The model under review builds one solid part; all positions refer to its coordinate system, in mm. Face numbers are marked on the shaded views. A direction names the side the tool comes from. Round coordinates to 2 decimals unless told otherwise and drop trailing zeros. Loops run counter-clockwise (first coordinate to the right, second up) from the corner with the lowest first, then second, coordinate; pieces in that order, holes last. Notation, with made-up numbers: M 17,83.5 L 36,83.5 A19 cw 36,94.5 Z; hole C 45,57 d10. An arc over 180 degrees is marked long. One line per question, with ' | ' between items.
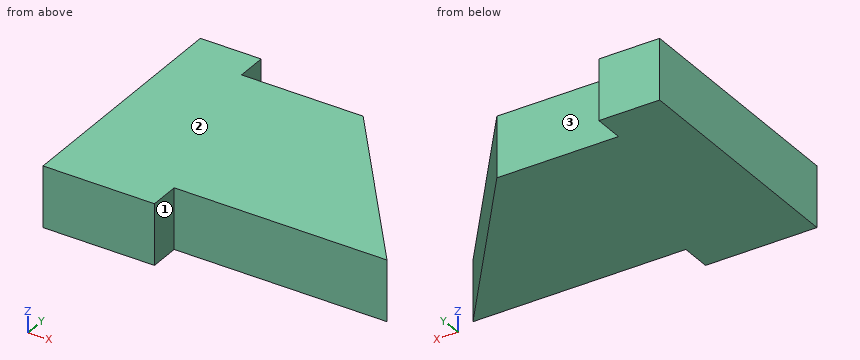
from build123d import *

# Parameters (mm, degrees)
EXTRUDE_1_DEPTH = 3
SKETCH_2_W      = 3
SKETCH_2_H      = 3
EXTRUDE_2_DEPTH = 1.5
SKETCH_3_W      = 5.5
SKETCH_3_H      = 3
EXTRUDE_3_DEPTH = 1.5


with BuildPart() as part:
    # Эскиз1 → Бобышка-Вытянуть1 (new body)
    with BuildSketch(Plane.XY):
        Polygon((0, 9), (0, 0), (16, 0), (9, 9), align=None)
    extrude(amount=EXTRUDE_1_DEPTH)

    # Эскиз2 → Бобышка-Вытянуть2 (add)
    with BuildSketch(Plane(origin=(0, 9, 0), x_dir=(1, 0, 0), z_dir=(0, 1, 0))):
        with Locations((1.5, -1.5)):
            Rectangle(SKETCH_2_W, SKETCH_2_H)
    extrude(amount=EXTRUDE_2_DEPTH)

    # Эскиз3 → Бобышка-Вытянуть3 (add)
    with BuildSketch(Plane.XZ):
        with Locations((2.75, 1.5)):
            Rectangle(SKETCH_3_W, SKETCH_3_H)
    extrude(amount=EXTRUDE_3_DEPTH)


solid = part.part
1) Machinability: for the marked faces 1, 2 and 3, which of the approach directions +Z, -Z, +X, -X, +Y, -Y give a long, thin tool a straight path to every point of the face, cutting with its end or side? Answer none if there is none.
Output values:
face 1: +Z, -Z, +X, -Y | face 2: +Z, +X, -X, +Y, -Y | face 3: +Z, -Z, +X, +Y
2) Add section A-A on z = 2.3. State the section outline as (x, y) points, then the cut area to 3 significant figures.
Output values:
outline: M 0,-1.5 L 5.5,-1.5 L 5.5,0 L 16,0 L 9,9 L 3,9 L 3,10.5 L 0,10.5 Z | area: 125 mm²
3) Add section B-B on x = 4. State the section outline as (y, z) points.
Output values:
outline: M -1.5,0 L 9,0 L 9,3 L -1.5,3 Z
4) For line 1 (X direction, y = 9.25, z = 2.85); line 2 (Y direction, x = 6.25, z = 2.3); line 3 (X direction, y = -0.75, z = 2.3), list the stretches that pass through material, from the lowest coordinate up.
Output values:
line 1: x = 0 to 3 | line 2: y = 0 to 9 | line 3: x = 0 to 5.5
5) Add section C-C on y = 6.25. State the section outline as (x, z) points.
Output values:
outline: M 0,0 L 11.14,0 L 11.14,3 L 0,3 Z
6) Insertion check: P1, Ø0.9, axis at x = 5.5, z = 1, coming from the +Y side; P2, Ø0.9, axis at x = 12, z = 2, coming from the -Y side; P3, Ø0.8, axis at y = 10, z = 1, coming from the +X side. Each pin has a flat end and moves straight along its axis. Give the tip position at first contact, or say it passes through.
Output values:
P1: stops at y = 9 | P2: stops at y = 0 | P3: stops at x = 3
